Can you work these out from the model? Positions are in its coordinate system, mm. A direction names the side the tool comes from. Give positions to 0.01 mm unless a question says otherwise; leave off trailing zeros. Loops run counter-clockwise (first coordinate to the right, second up) from the corner with the lowest first, then second, coordinate; pieces in that order, holes last. Notation, with made-up numbers: (-40, 65.5) - (9, 65.5) arc R22 cw to (9, 98.5) - close; hole circle Ø8 at (24.5, -13). An arc over 180 degrees is marked (long way). Answer as a JSON object with one key per item and string values.
```python
from build123d import *

# Parameters (mm, degrees)
SKETCH1_R           = 25
SKETCH1_R_2         = 1
SKETCH1_R_3         = 2
BOSS_EXTRUDE1_DEPTH = 5
SKETCH2_W           = 5
SKETCH2_H           = 3
BOSS_EXTRUDE2_DEPTH = 20
SKETCH3_R           = 1
CUT_EXTRUDE1_DEPTH  = 57.444663167


with BuildPart() as part:
    # Sketch1 → Boss-Extrude1 (new body)
    with BuildSketch(Plane.XY):
        Circle(SKETCH1_R)
        with Locations((0, 8)):
            Circle(SKETCH1_R_2, mode=Mode.SUBTRACT)
        with Locations((8, 0)):
            Circle(SKETCH1_R_2, mode=Mode.SUBTRACT)
        with Locations((0, -8)):
            Circle(SKETCH1_R_2, mode=Mode.SUBTRACT)
        with Locations((-8, 0)):
            Circle(SKETCH1_R_2, mode=Mode.SUBTRACT)
        Circle(SKETCH1_R_3, mode=Mode.SUBTRACT)
    extrude(amount=BOSS_EXTRUDE1_DEPTH)

    # Sketch2 → Boss-Extrude2 (add)
    with BuildSketch(Plane.XY.offset(5)):
        with Locations((-13.5, 17.5)):
            Rectangle(SKETCH2_W, SKETCH2_H)
        with Locations((13.5, 17.5)):
            Rectangle(SKETCH2_W, SKETCH2_H)
        with Locations((-13.5, -17.5)):
            Rectangle(SKETCH2_W, SKETCH2_H)
        with Locations((13.5, -17.5)):
            Rectangle(SKETCH2_W, SKETCH2_H)
    extrude(amount=BOSS_EXTRUDE2_DEPTH)

    # Sketch3 → Cut-Extrude1 (cut, through all)
    with BuildSketch(Plane.XZ.offset(19)):
        with Locations(Location((-13.5, 20.75, 0), (0, 0, 270))):
            Circle(SKETCH3_R)
        with Locations(Location((-13.5, 12.75, 0), (0, 0, 270))):
            Circle(SKETCH3_R)
        with Locations(Location((13.5, 20.75, 0), (0, 0, 180))):
            Circle(SKETCH3_R)
        with Locations(Location((13.5, 12.75, 0), (0, 0, 180))):
            Circle(SKETCH3_R)
    extrude(amount=-CUT_EXTRUDE1_DEPTH, mode=Mode.SUBTRACT)


solid = part.part
```
1) Imagine slicing it at D-D on x = 13.5. Write out the boundary of the cut face in (y, z).
Check sheet entries:
{"outline": "(-21.04, 0) - (21.04, 0) - (21.04, 5) - (19, 5) - (19, 11.75) - (16, 11.75) - (16, 5) - (-16, 5) - (-16, 11.75) - (-19, 11.75) - (-19, 5) - (-21.04, 5) - close; (-19, 13.75) - (-16, 13.75) - (-16, 19.75) - (-19, 19.75) - close; (-19, 21.75) - (-16, 21.75) - (-16, 25) - (-19, 25) - close; (16, 13.75) - (19, 13.75) - (19, 19.75) - (16, 19.75) - close; (16, 21.75) - (19, 21.75) - (19, 25) - (16, 25) - close"}
2) Imagine slicing it at B-B on z = 18.5. Write out the boundary of the cut face in (x, y), and give its area (3 significant figures).
Check sheet entries:
{"outline": "(-16, -19) - (-11, -19) - (-11, -16) - (-16, -16) - close; (-16, 16) - (-11, 16) - (-11, 19) - (-16, 19) - close; (11, -19) - (16, -19) - (16, -16) - (11, -16) - close; (11, 16) - (16, 16) - (16, 19) - (11, 19) - close", "area": "60.0 mm2"}
3) Imagine slicing it at C-C on y = -8. Write out the boundary of the cut face in (x, z), and give its area (3 significant figures).
Check sheet entries:
{"outline": "(-23.69, 0) - (-1, 0) - (-1, 5) - (-23.69, 5) - close; (1, 0) - (23.69, 0) - (23.69, 5) - (1, 5) - close", "area": "227 mm2"}
4) I need wall thicknesses on L1, parallel to X at y = 18, z = 20.75; L2, parallel to Z at x = 13.5, y = 18.15; L3, parallel to Y at x = -13.5, z = 18.25. Which ranges of each line are inside material? Lowest first, please.
Check sheet entries:
{"L1": "-16 to -14.5, -12.5 to -11, 11 to 12.5, 14.5 to 16", "L2": "0 to 11.75, 13.75 to 19.75, 21.75 to 25", "L3": "-19 to -16, 16 to 19"}
5) If we mould it in two halves opening along X, with no side actions, what happens to faces 1 (the flat face through (16, -18, 15)), 2 (the flat face through (-14, 18, 25)), 3 (the cylindrical face through (0, -7, 2))? For each: released by +X, released by -X, zero draft, split by the parting line, or undercut.
Check sheet entries:
{"face 1": "released by +X", "face 2": "zero draft", "face 3": "undercut"}
6) Imagine slicing it at A-A on y = 0. Write out the boundary of the cut face in (x, z), and give its area (3 significant figures).
Check sheet entries:
{"outline": "(-25, 0) - (-9, 0) - (-9, 5) - (-25, 5) - close; (-7, 0) - (-2, 0) - (-2, 5) - (-7, 5) - close; (2, 0) - (7, 0) - (7, 5) - (2, 5) - close; (9, 0) - (25, 0) - (25, 5) - (9, 5) - close", "area": "210 mm2"}
7) Which directions (+Z, -Z, +X, -X, +Y, -Y) give clear straight access to the entire face, cutting with the end or side of a thin tool? Please do faces 4 (the flat face through (-11, 17, 15)), 5 (the flat face through (13, -16, 15)), 6 (the flat face through (13, -19, 15)), 7 (the flat face through (13, 19, 15)).
Check sheet entries:
{"face 4": "+Z, +Y, -Y", "face 5": "+Z, +X, -X", "face 6": "+Z, +X, -X, -Y", "face 7": "+Z, +X, -X, +Y"}
8) I'm going to push flat-ended pins straight in: P1, Ø2.5, axis at x = -13.5, z = 20.75, coming from the -Y side; P2, Ø2.5, axis at y = -17.5, z = 11.5, coming from the +X side; P3, Ø12, axis at x = -8, z = 12, coming from the +Y side; P4, Ø1.8, axis at x = 13.5, z = 12.75, coming from the -Y side. Where does each tip first touch, or does it pass through?
Check sheet entries:
{"P1": "y = -19", "P2": "x = 16", "P3": "y = 19", "P4": "through"}
